Check sheet for the modelled part. Datum: model origin and axes. Units: mm. A direction names the side the tool comes from. Give positions to 0.01 mm unless a question says otherwise; leave off trailing zeros. Write each question's results on one line, items separated by ' | '. Start each with the question number.
1. Gauge pin test, flat ends, axial feed: pin 1 Ø0.8 at (x, y) = (1, 12) entering from -Z; pin 2 Ø0.5 at (x, z) = (0.5, -13.5) entering from +Y. Record the tip position at first contact, or that the pin passes through.
2. Material ranges on L1, parallel to Z at x = 1.3, y = -18.5; L2, parallel to X at y = -18, z = 2.5; L3, parallel to Z at x = 0.2, y = 18, recorded low to high. Write a range as from..to.
3. Tool access check on faces 1 (the face through (1, 18, -12.7)), 2 (the face through (1, -18, -12.7)), 3 (the face through (1, 0, -14.288)). Record the directions out of +Z, -Z, +X, -X, +Y, -Y that give a thin tool (end or side, any length) a straight path to the whole face; none if there is none.
from build123d import *
from OCP.BRepAlgoAPI import BRepAlgoAPI_Cut
from OCP.TopTools import TopTools_ListOfShape

# Parameters (mm, degrees)
SKETCH2_W           = 25.4
SKETCH2_H           = 63.5
BOSS_EXTRUDE1_DEPTH = 1.5875
SKETCH3_W           = 1.5875
SKETCH3_H           = 9.525
BOSS_EXTRUDE2_DEPTH = 1.5875
SKETCH3_4_W         = 1.5875
SKETCH3_4_H         = 9.525
CUT_EXTRUDE1_DEPTH  = 3.175
CUT_EXTRUDE2_DEPTH  = 35.85276621
CAVITY1_START       = -31.74999873
CAVITY1_DEPTH       = 63.499999998


with BuildPart() as part:
    # Sketch2 → Boss-Extrude1 (new body)
    with BuildSketch(Plane(origin=(0, 0, 0), x_dir=(0, 0, -1), z_dir=(1, 0, 0))):
        Rectangle(SKETCH2_W, SKETCH2_H)
    extrude(amount=BOSS_EXTRUDE1_DEPTH)

    # Sketch3 → Boss-Extrude2 (add)
    with BuildSketch(Plane(origin=(1.5875, 0, 0), x_dir=(0, 0, -1), z_dir=(1, 0, 0))):
        with Locations((13.49375, 0)):
            Rectangle(SKETCH3_W, SKETCH3_H)
    extrude(amount=-BOSS_EXTRUDE2_DEPTH)

    # Sketch3<4> → Cut-Extrude1 (cut)
    with BuildSketch(Plane(origin=(1.5875, 0, 0), x_dir=(0, 0, -1), z_dir=(1, 0, 0))):
        with Locations((-11.90625, 0)):
            Rectangle(SKETCH3_4_W, SKETCH3_4_H)
    extrude(amount=-CUT_EXTRUDE1_DEPTH, mode=Mode.SUBTRACT)

    # Sketch4 → Cut-Extrude2 (cut, through all)
    with BuildSketch(Plane(origin=(1.5875, 0, 0), x_dir=(0, 0, -1), z_dir=(1, 0, 0))):
        Polygon((-6.14934, 31.75), (-6.14934, -31.75), (-12.7, -31.75), (-12.7, -4.7625), (-11.1125, -4.7625), (-11.1125, 4.7625), (-12.7, 4.7625), (-12.7, 31.75), align=None)
    extrude(amount=-CUT_EXTRUDE2_DEPTH, mode=Mode.SUBTRACT)


with BuildPart() as cavity1_tool:
    # Cavity1: read off the stored shape, not the designer's step
    # Cavity1 outline → Cavity1 (new body)
    with BuildSketch(Plane(origin=(0, 0, 0), x_dir=(0.9999999999641164, -8.471563968881495e-06, 0), z_dir=(8.471563968881494e-06, 0.9999999999641164, 0)).offset(CAVITY1_START)):
        with BuildLine():
            Line((-2, -6.14934), (1.17475, -6.14934))
            ThreePointArc((1.17475, -6.14934), (0.877620674, -3.377118582), (-0.000268972, -0.730836814))
            Line((-0.000268972, -0.730836814), (-0.787986067, 1))
            Line((-0.787986067, 1), (-2, 1))
            Line((-2, 1), (-2, -6.14934))
        make_face()
    extrude(amount=CAVITY1_DEPTH)


with BuildPart() as part_1:
    add(part.part)

    # Cavity1: cut by cavity1_tool, with a tolerance
    cavity1_stock = TopTools_ListOfShape()
    cavity1_stock.Append(part_1.part.wrapped)
    cavity1_tools = TopTools_ListOfShape()
    cavity1_tools.Append(cavity1_tool.part.wrapped)
    cavity1_cut = BRepAlgoAPI_Cut()
    cavity1_cut.SetArguments(cavity1_stock)
    cavity1_cut.SetTools(cavity1_tools)
    cavity1_cut.SetFuzzyValue(0.00001)
    cavity1_cut.Build()
    add(Compound.cast(cavity1_cut.Shape()).solids(), mode=Mode.REPLACE)


solid = part_1.part
Geometry says:
1) pin 1: z = -12.7 | pin 2: y = 4.76
2) L1: -12.7..6.15 | L2: 0.66..1.59 | L3: -12.7..1.19
3) face 1: -Z, +X, -X, +Y | face 2: -Z, +X, -X, -Y | face 3: -Z, +X, -X, +Y, -Y
